For this review, use the dimensioned drawing (mm, ordinates from the lowest corner) and the shaded views. A direction names the side the tool comes from. Give positions to 0.01 mm unless a question says otherwise; leave off trailing zeros. Loops run counter-clockwise (first coordinate to the right, second up) from the corner with the lowest first, then second, coordinate; pieces in that order, holes last. Notation, with made-up numbers: M 50,-21.5 L 99,-21.5 A26 cw 99,9.5 Z; hole C -20,17 d10. An arc over 180 degrees is marked long. Use a Markdown table: item, result. Add a question column.
(1) Add section B-B, the plane x = 5.1. Give the boundary of the cut face in (y, z).
(2) Insertion check: pin 1 Ø0.8 at (x, z) = (1, 6) entering from +Y; pin 2 Ø0.7 at (y, z) = (4.5, 5.5) entering from +X; pin 3 Ø1.5 at (x, z) = (1.5, 1.5) entering from +Y. Each pin has a flat end and moves straight along its axis. Give the tip position at first contact, or say it passes through.
(3) Add section C-C, the plane z = 9. Give the boundary of the cut face in (x, y).
(4) For the marked faces 1, 2 and 3, list the 3-axis set-ups (+Z, -Z, +X, -X, +Y, -Y) from which the entire face can be reached by the end or side of a thin tool; tool diameter is ignored.
(5) For probe 1 along X at (y, z) = (2.25, 5.5); probe 2 along X at (y, z) = (4.65, 0.5); probe 3 along X at (y, z) = (0.2, 6.75), list the stretches that pass through material, from the lowest coordinate up.
(6) Add section D-D, the plane x = 6.5. Give the boundary of the cut face in (y, z).
(7) Add section A-A, the plane z = 5.5. Give the boundary of the cut face in (x, y).
(8) Draft analysis for pull direction Z (two halves, no side actions). For the marked faces 4, 5 and 6, state which applies: pulls with the +Z half, pulls with the -Z half, needs draft (parallel to the pull), parting line crosses it, or undercut.
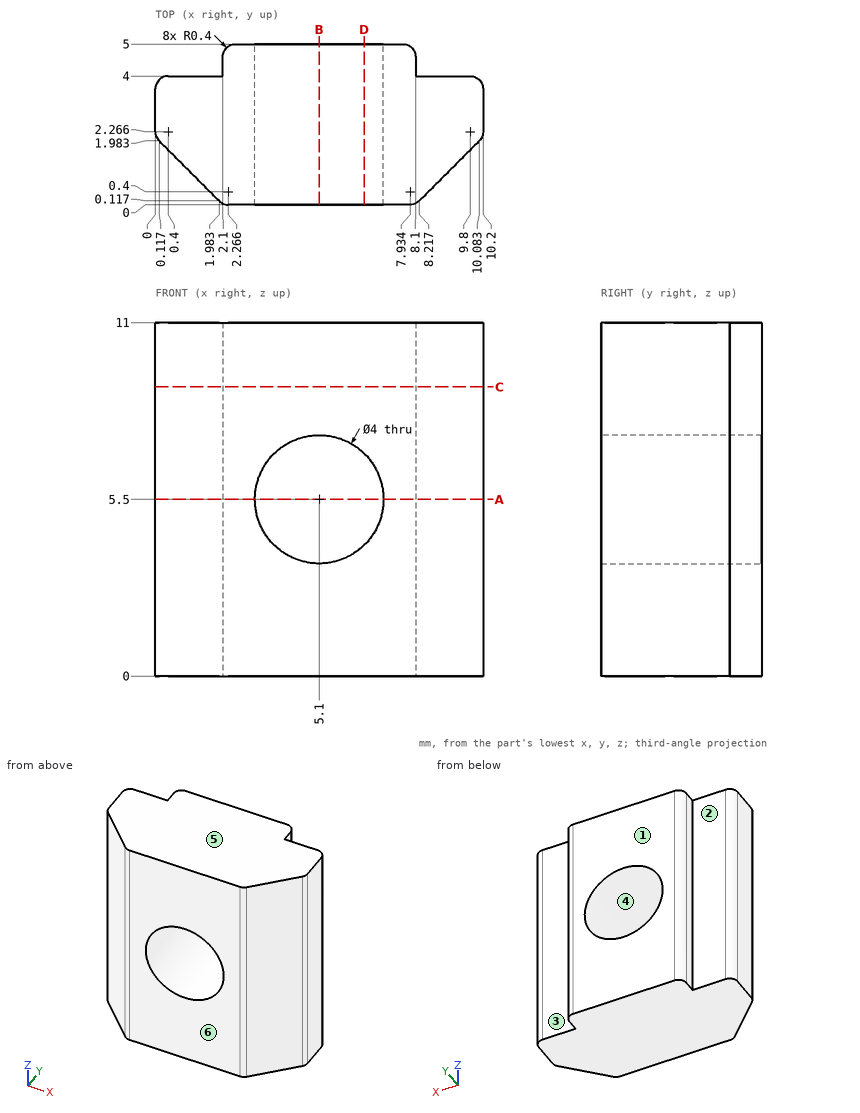
Established:
| question | item | result |
|---|---|---|
| 1 | outline | M 0,0 L 5,0 L 5,3.5 L 0,3.5 Z; M 0,7.5 L 5,7.5 L 5,11 L 0,11 Z |
| 2 | pin 1 | y = 4 |
| 2 | pin 2 | x = 8.1 |
| 2 | pin 3 | y = 4.91 |
| 3 | outline | M 0,2.27 A0.4 ccw 0.12,1.98 L 1.98,0.12 A0.4 ccw 2.27,0 L 7.93,0 A0.4 ccw 8.22,0.12 L 10.08,1.98 A0.4 ccw 10.2,2.27 L 10.2,3.6 A0.4 ccw 9.8,4 L 8.1,4 L 8.1,4.6 A0.4 ccw 7.7,5 L 2.5,5 A0.4 ccw 2.1,4.6 L 2.1,4 L 0.4,4 A0.4 ccw 0,3.6 Z |
| 4 | face 1 | +Z, -Z, +X, -X, +Y |
| 4 | face 2 | +Z, -Z, -X, +Y |
| 4 | face 3 | +Z, -Z, +X, +Y |
| 5 | probe 1 | 0 to 3.1, 7.1 to 10.2 |
| 5 | probe 2 | 2.1 to 8.1 |
| 5 | probe 3 | 1.9 to 3.54, 6.66 to 8.3 |
| 6 | outline | M 0,0 L 5,0 L 5,4.07 L 0,4.07 Z; M 0,6.93 L 5,6.93 L 5,11 L 0,11 Z |
| 7 | outline | M 0,2.27 A0.4 ccw 0.12,1.98 L 1.98,0.12 A0.4 ccw 2.27,0 L 3.1,0 L 3.1,5 L 2.5,5 A0.4 ccw 2.1,4.6 L 2.1,4 L 0.4,4 A0.4 ccw 0,3.6 Z; M 7.1,0 L 7.93,0 A0.4 ccw 8.22,0.12 L 10.08,1.98 A0.4 ccw 10.2,2.27 L 10.2,3.6 A0.4 ccw 9.8,4 L 8.1,4 L 8.1,4.6 A0.4 ccw 7.7,5 L 7.1,5 Z |
| 8 | face 4 | undercut |
| 8 | face 5 | pulls with the +Z half |
| 8 | face 6 | needs draft |
